Model file for the job. Use its own axes, mm. A direction names the side the tool comes from. Coordinates: 2 decimals unless noted, no trailing zeros. Order: outer loops, then holes, each group sorted by start corner. A loop starts at its lowest first (then second) coordinate and runs counter-clockwise, first axis right, second up.
from build123d import *

# Parameters (mm, degrees)
SKETCH1_R           = 34
SKETCH1_R_2         = 32
BOSS_EXTRUDE1_DEPTH = 12
BOSS_EXTRUDE2_START = -2
SKETCH2_R           = 34
BOSS_EXTRUDE2_DEPTH = 2
SKETCH3_R           = 10
SKETCH3_R_2         = 8.5
BOSS_EXTRUDE3_DEPTH = 7


with BuildPart() as part:
    # Sketch1 → Boss-Extrude1 (new body)
    with BuildSketch(Plane.XY):
        Circle(SKETCH1_R)
        Circle(SKETCH1_R_2, mode=Mode.SUBTRACT)
    extrude(amount=BOSS_EXTRUDE1_DEPTH)

    # Sketch2 → Boss-Extrude2 (add)
    with BuildSketch(Plane.XY.offset(12).offset(BOSS_EXTRUDE2_START)):
        Circle(SKETCH2_R)
    extrude(amount=BOSS_EXTRUDE2_DEPTH)

    # Sketch3 → Boss-Extrude3 (add)
    with BuildSketch(Plane(origin=(0, 0, 10), x_dir=(-1, 0, 0), z_dir=(0, 0, -1))):
        with Locations(Location((0, 0, 0), (0, 0, 180))):
            Circle(SKETCH3_R)
        Circle(SKETCH3_R_2, mode=Mode.SUBTRACT)
    extrude(amount=BOSS_EXTRUDE3_DEPTH)


solid = part.part
Q1. Cut at D-D, the plane y = -12. List the corners of the cut face in (x, z), plus the area to 3 significant figures.
Established:
outline: (-31.81, 0) - (-29.66, 0) - (-29.66, 10) - (29.66, 10) - (29.66, 0) - (31.81, 0) - (31.81, 12) - (-31.81, 12) - close
area: 170 mm2
Q2. Probe line 1 (Y direction, x = 0, z = 7); line 2 (Z direction, x = -11, y = 12); line 3 (Y direction, x = 4, z = 6.5). List the from-to ranges inside material, lowest first.
Established:
line 1: y = -34 to -32, -10 to -8.5, 8.5 to 10, 32 to 34
line 2: z = 10 to 12
line 3: y = -33.76 to -31.75, -9.17 to -7.5, 7.5 to 9.17, 31.75 to 33.76
Q3. Drop flat-ended pins along their axis: P1, Ø19, axis at x = -7.5, y = -6.5, coming from the -Z side; P2, Ø6, axis at x = 6.5, z = 6, coming from the -Y side; P3, Ø2, axis at x = 2, y = 22, coming from the -Z side. Give the stop position or say it passes through.
Established:
P1: stops at z = 3
P2: stops at y = -33.82
P3: stops at z = 10
Q4. Cut at A-A, the plane z = 5. List the corners of the cut face in (x, y), plus the area to 3 significant figures.
Established:
outline: circle Ø68 at (0, 0); circle Ø20 at (0, 0); hole circle Ø64 at (0, 0); hole circle Ø17 at (0, 0)
area: 502 mm2
Q5. Cut at B-B, the plane y = 0. List the corners of the cut face in (x, z).
Established:
outline: (-34, 0) - (-32, 0) - (-32, 10) - (-10, 10) - (-10, 3) - (-8.5, 3) - (-8.5, 10) - (8.5, 10) - (8.5, 3) - (10, 3) - (10, 10) - (32, 10) - (32, 0) - (34, 0) - (34, 12) - (-34, 12) - close
Q6. Mould opens along X. For faces 1 (the face through (-23, -23, 0)), 2 (the face through (0, 0, 10)), 3 (the face through (-4.57, 7.167, 6.549)), 4 (the face through (18.28, 28.67, 5.92)) say: pulls with the +X half, pulls with the -X half, needs draft (parallel to the pull), parting line crosses it, or undercut.
Established:
face 1: needs draft
face 2: undercut
face 3: undercut
face 4: parting line crosses it
Q7. Which spindle directions (+Z, -Z, +X, -X, +Y, -Y) get a long thin tool onto all of the face, cutting with end or side? Do faces 5 (the face through (0, 0, 12)), 6 (the face through (-4.5, 7.4, 3)). Say none if no direction does.
Established:
face 5: +Z, +X, -X, +Y, -Y
face 6: -Z
